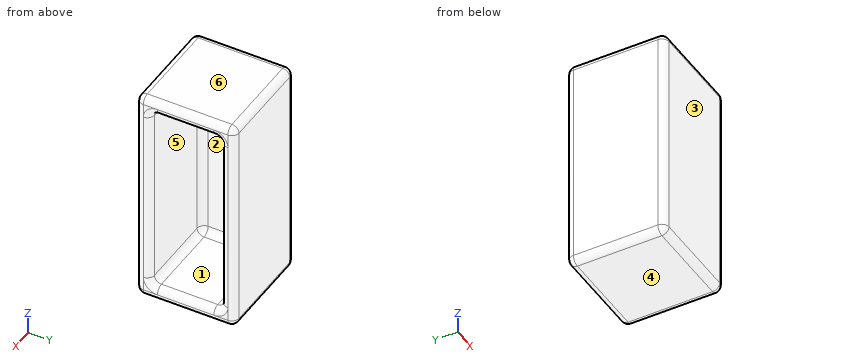
from build123d import *

# Parameters (mm, degrees)
F0_W     = 18.5276605189
F0_H     = 39.9128235877
F1_DEPTH = 17.78
F2_T     = -2.54
F3_R     = 1.26999


# Not quite as in the source:
# - a fillet or chamfer is up to 0.001 mm smaller than in the source, because OpenCascade refuses the exact size


with BuildPart() as f1:
    # F0 (on Front) → F1 (new body)
    with BuildSketch(Plane.XZ):
        with Locations((9.2638302594, 19.9564117938)):
            Rectangle(F0_W, F0_H)
    extrude(amount=F1_DEPTH)

    # F2
    f2_openings = [f1.faces().sort_by_distance(p)[0] for p in [
        (18.527661, -8.89, 19.956412),
    ]]
    offset(amount=F2_T, openings=f2_openings)

    # F3 (radius 1.27 in the source; OpenCascade refuses exactly that, so slightly less here)
    f3_edges = [f1.edges().sort_by_distance(p)[0] for p in [
        (18.527661, 0, 19.956412),
        (18.527661, -2.54, 19.956412),
        (18.527661, -8.89, 37.372824),
        (18.527661, -8.89, 39.912824),
        (18.527661, -15.24, 19.956412),
        (18.527661, -17.78, 19.956412),
        (18.527661, -8.89, 2.54),
        (18.527661, -8.89, 0),
        (9.26383, 0, 39.912824),
        (0, -8.89, 39.912824),
        (9.26383, -17.78, 39.912824),
        (2.54, -15.24, 19.956412),
        (2.54, -8.89, 2.54),
        (0, 0, 19.956412),
        (9.26383, 0, 0),
        (0, -17.78, 19.956412),
        (0, -8.89, 0),
        (9.26383, -17.78, 0),
        (2.54, -2.54, 19.956412),
        (10.53383, -2.54, 37.372824),
        (2.54, -8.89, 37.372824),
        (10.53383, -2.54, 2.54),
        (10.53383, -15.24, 2.54),
        (10.53383, -15.24, 37.372824),
    ]]
    fillet(f3_edges, radius=F3_R)


solid = f1.part
Input: part model. Units: mm. Frame: model coordinates. Face numbers are marked on the shaded views. A direction names the side the tool comes from. Round coordinates to 2 decimals unless told otherwise and drop trailing zeros. Loops run counter-clockwise (first coordinate to the right, second up) from the corner with the lowest first, then second, coordinate; pieces in that order, holes last. Notation, with made-up numbers: (51.25, 0.25) -> (80.25, 0.25) arc R30 ccw to (80.25, 34.25) -> close; hole circle Ø10 at (8, 27.5). An arc over 180 degrees is marked (long way). Answer as a JSON object with one key per item and string values. Group by question number.
1) Ray query, L1, parallel to Y at x = 9, z = 35; L2, parallel to Z at x = 9.75, y = -5.75; L3, parallel to X at y = -13.5, z = 8. Return the intervals inside material, ascending.
2) Draft query along Z for the marked faces 1, 2, 3 and 4. Return one class per face: +Z half, -Z half, draft (parallel to the pull), parting line (faces both ways), or undercut.
3) Reachability of the marked faces 5 and 6 from +Z, -Z, +X, -X, +Y, -Y: full face, straight path, thin tool, end or side. Return the list, or none.
4) Section query B-B on x = 14.25. Output: boundary loops of the cut face in (y, z).
5) Pin query (flat end, axial travel): pin 1 (1 mm diameter, centred on y = -12.5, z = 19.5, fed in from +X). Return the tip coordinate at first contact, or that it passes through.
Reply:
{
 "1": {"L1": "y = -17.78 to -15.24, -2.54 to 0", "L2": "z = 0 to 2.54, 37.37 to 39.91", "L3": "x = 0 to 2.54"},
 "2": {"face 1": "undercut", "face 2": "undercut", "face 3": "draft", "face 4": "-Z half"},
 "3": {"face 5": "+X", "face 6": "+Z, +X, -X, +Y, -Y"},
 "4": {"outline": "(-17.78, 1.27) arc R1.27 ccw to (-16.51, 0) -> (-1.27, 0) arc R1.27 ccw to (0, 1.27) -> (0, 38.64) arc R1.27 ccw to (-1.27, 39.91) -> (-16.51, 39.91) arc R1.27 ccw to (-17.78, 38.64) -> close; hole (-15.24, 3.81) arc R1.27 ccw to (-13.97, 2.54) -> (-3.81, 2.54) arc R1.27 ccw to (-2.54, 3.81) -> (-2.54, 36.1) arc R1.27 ccw to (-3.81, 37.37) -> (-13.97, 37.37) arc R1.27 ccw to (-15.24, 36.1) -> close"},
 "5": {"pin 1": "stops at x = 2.54"}
}
